Part model, mm, in its own coordinate system. Face numbers are marked on the shaded views. A direction names the side the tool comes from. Round coordinates to 2 decimals unless told otherwise and drop trailing zeros. Loops run counter-clockwise (first coordinate to the right, second up) from the corner with the lowest first, then second, coordinate; pieces in that order, holes last.
(1) Mould opens along Z. For the marked faces 1, 2 and 3 say: +Z half, -Z half, draft (parallel to the pull), parting line (faces both ways), or undercut.
(2) Cut at A-A on z = 7. List the corners of the cut face in (x, y).
(3) Cut at B-B on z = 27.5. List the corners of the cut face in (x, y).
(4) Tool access for the marked faces 4, 5 and 6: list every direction of +Z, -Z, +X, -X, +Y, -Y with a clear straight run to the whole face (end or side of a thin tool).
(5) Probe probe 1 along Y at (x, z) = (20, 17); probe 2 along Z at (x, y) = (4, -11.5); probe 3 along X at (y, z) = (0, 13.25). List the from-to ranges inside material, lowest first.
(6) Flat gauge pins, fed straight in: pin 1 (4 mm diameter, centred on x = 22.5, y = -2, fed in from -Z); pin 2 (2 mm diameter, centred on y = 3, z = 30, fed in from -X); pin 3 (5.5 mm diameter, centred on x = 38, z = 7, fed in from +Y); pin 4 (9 mm diameter, centred on x = 20, y = 0, fed in from -Z). Where does each tip first touch, or does it go through?
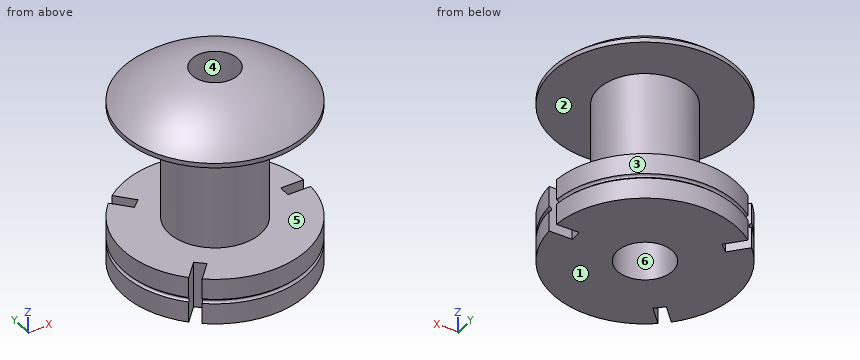
from build123d import *

# Parameters (mm, degrees)
F2_R     = 5
F3_DEPTH = 43.9649
F4_R     = 6
F5_DEPTH = 25


with BuildPart() as f1:
    # F0 (on Front) → F1 (revolve)
    with BuildSketch(Plane.XZ):
        with BuildLine():
            Line((0, 4.5), (0, 0))
            Line((0, 0), (20, 0))
            Line((20, 0), (20, 43.964899))
            ThreePointArc((20, 43.964899), (9.236176, 41.900424), (0, 36))
            Line((0, 36), (0, 35))
            Line((0, 35), (10, 35))
            Line((10, 35), (10, 10))
            Line((10, 10), (0, 10))
            Line((0, 10), (0, 5.5))
            ThreePointArc((0, 5.5), (0.353553, 5.353553), (0.5, 5))
            ThreePointArc((0.5, 5), (0.353553, 4.646447), (0, 4.5))
        make_face()
    revolve(axis=Axis((20, 0, 21.982449), (0, 0, 1)))

    # F2 (on face) → F3 (cut)
    with BuildSketch(Plane(origin=(0, 0, 0), x_dir=(1, 0, 0), z_dir=(0, 0, -1))):
        with Locations((20, 0)):
            Circle(F2_R)
    extrude(amount=-F3_DEPTH, mode=Mode.SUBTRACT)

    # F4 (on face) → F5 (cut)
    with BuildSketch(Plane(origin=(0, 0, 0), x_dir=(1, 0, 0), z_dir=(0, 0, -1))):
        with Locations((20, 0)):
            Circle(F4_R)
        Polygon((8.944216, 10.214311), (10.787355, 11.903347), (6.733669, 16.326878), (4.890531, 14.637843), align=None)
        Polygon((35.039323, -1.249084), (41.039323, -1.249084), (40.971649, 1.25), (34.971649, 1.25), align=None)
        Polygon((9.032436, -10.308979), (5.016928, -14.767196), (6.874519, -16.440324), (10.890026, -11.982107), align=None)
    extrude(amount=-F5_DEPTH, mode=Mode.SUBTRACT)


solid = f1.part
Final values:
1. face 1: -Z half
1. face 2: undercut
1. face 3: draft
2. outline: (5.59, -13.87) - (8.94, -10.21) - (10.79, -11.9) - (7.44, -15.56) arc R20 ccw to (39.96, -1.25) - (34.97, -1.25) - (35.04, 1.25) - (39.96, 1.25) arc R20 ccw to (7.57, 15.67) - (10.89, 11.98) - (9.03, 10.31) - (5.71, 14) arc R20 ccw to start; hole circle Ø12 at (20, 0)
3. outline: circle Ø20 at (20, 0); hole circle Ø10 at (20, 0)
4. face 4: +Z, -Z
4. face 5: none
4. face 6: -Z
5. probe 1: y = -10 to -6, 6 to 10
5. probe 2: z = 0 to 4.6, 5.4 to 10, 35 to 36.28
5. probe 3: x = 10 to 14, 26 to 30
6. pin 1: stops at z = 25
6. pin 2: stops at x = 10.2
6. pin 3: stops at y = 12.94
6. pin 4: passes through
